The figure shows three views and two pictorial views of one solid part (mm, origin at its lowest corner). Answer the questions. A direction names the side the tool comes from. Coordinates: 2 decimals unless noted, no trailing zeros. Order: outer loops, then holes, each group sorted by start corner. A loop starts at its lowest first (then second) coordinate and runs counter-clockwise, first axis right, second up. Notation, with made-up numbers: (-9, 0) -> (13, 0) arc R21 cw to (13, 6) -> close; hole circle Ø9 at (7.5, -23). An arc over 180 degrees is marked (long way). Return JSON: item names as keys, results as strings.
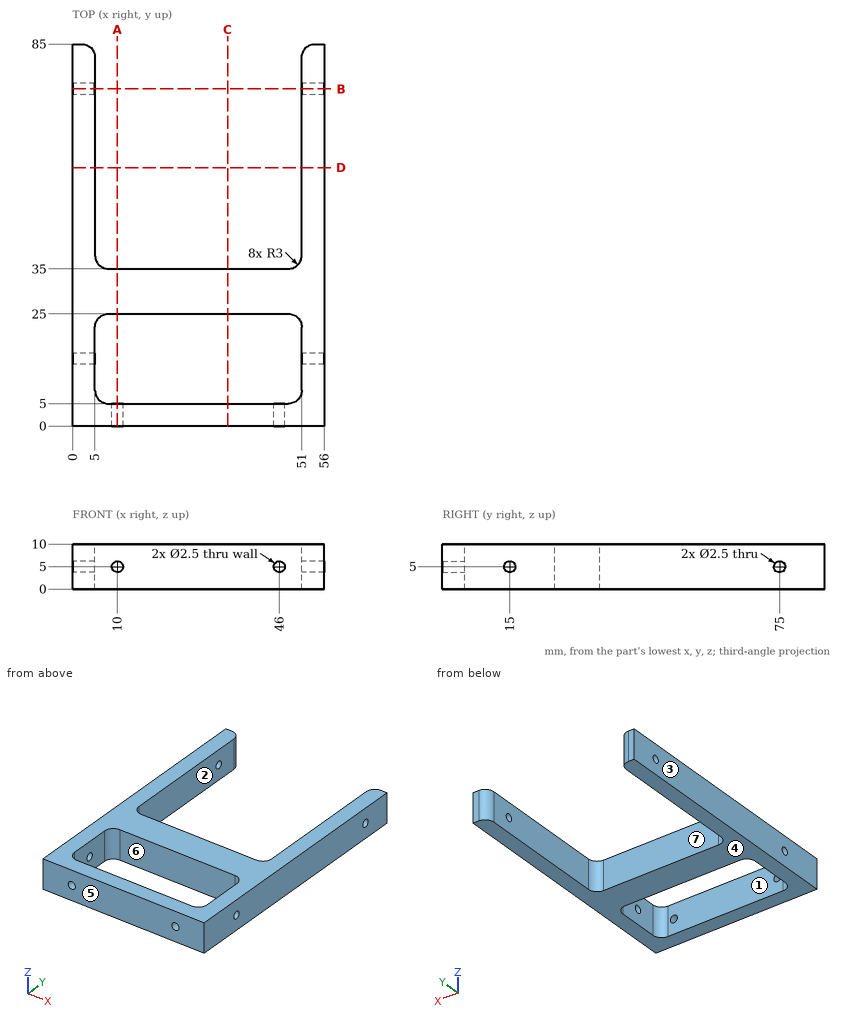
Item 1: Determine the mould class of the marked faces 4, 5, 6 and 7 for opening direction Y: pulls with the +Y half, pulls with the -Y half, needs draft (parallel to the pull), parting line crosses it, or undercut.
Answer list:
{"face 4": "needs draft", "face 5": "pulls with the -Y half", "face 6": "undercut", "face 7": "pulls with the +Y half"}
Item 2: The part is cut by section D-D on y = 57.5. Determine the outline of the cut face in (x, z).
Answer list:
{"outline": "(0, 0) -> (5, 0) -> (5, 10) -> (0, 10) -> close; (51, 0) -> (56, 0) -> (56, 10) -> (51, 10) -> close"}
Item 3: The part is cut by section A-A on x = 10. Determine the outline of the cut face in (y, z).
Answer list:
{"outline": "(0, 0) -> (5, 0) -> (5, 3.75) -> (0, 3.75) -> close; (0, 6.25) -> (5, 6.25) -> (5, 10) -> (0, 10) -> close; (25, 0) -> (35, 0) -> (35, 10) -> (25, 10) -> close"}
Item 4: The part is cut by section B-B on y = 75. Determine the outline of the cut face in (x, z), plus the area to 3 significant figures.
Answer list:
{"outline": "(0, 0) -> (5, 0) -> (5, 3.75) -> (0, 3.75) -> close; (0, 6.25) -> (5, 6.25) -> (5, 10) -> (0, 10) -> close; (51, 0) -> (56, 0) -> (56, 3.75) -> (51, 3.75) -> close; (51, 6.25) -> (56, 6.25) -> (56, 10) -> (51, 10) -> close", "area": "75.0 mm2"}
Item 5: The part is cut by section C-C on x = 34.5. Determine the outline of the cut face in (y, z), plus the area to 3 significant figures.
Answer list:
{"outline": "(0, 0) -> (5, 0) -> (5, 10) -> (0, 10) -> close; (25, 0) -> (35, 0) -> (35, 10) -> (25, 10) -> close", "area": "150 mm2"}
Item 6: Which of the six approach directions +Z, -Z, +X, -X, +Y, -Y give full straight-line access (tool end or side, diameter ignored) to the marked faces 1, 2 and 3?
Answer list:
{"face 1": "+Z, -Z", "face 2": "+Z, -Z, +Y", "face 3": "+Z, -Z, -X, +Y, -Y"}
Item 7: Flat-ended cylindrical pins translate along their axes: pin 1 (1.5 mm diameter, centred on x = 28, z = 4.5, fed in from +Y); pin 2 (1.5 mm diameter, centred on x = 46, z = 5, fed in from -Y). Find the tip coordinate at first contact, or state that the pin passes through.
Answer list:
{"pin 1": "y = 35", "pin 2": "y = 25"}
Item 8: Find the intervals of material crossed by probe 1 along X at (y, z) = (3.4, 5); probe 2 along Y at (x, z) = (54.4, 5); probe 3 along Y at (x, z) = (13, 9), in increasing order.
Answer list:
{"probe 1": "0 to 8.75, 11.25 to 44.75, 47.25 to 56", "probe 2": "0 to 13.75, 16.25 to 73.75, 76.25 to 85", "probe 3": "0 to 5, 25 to 35"}
